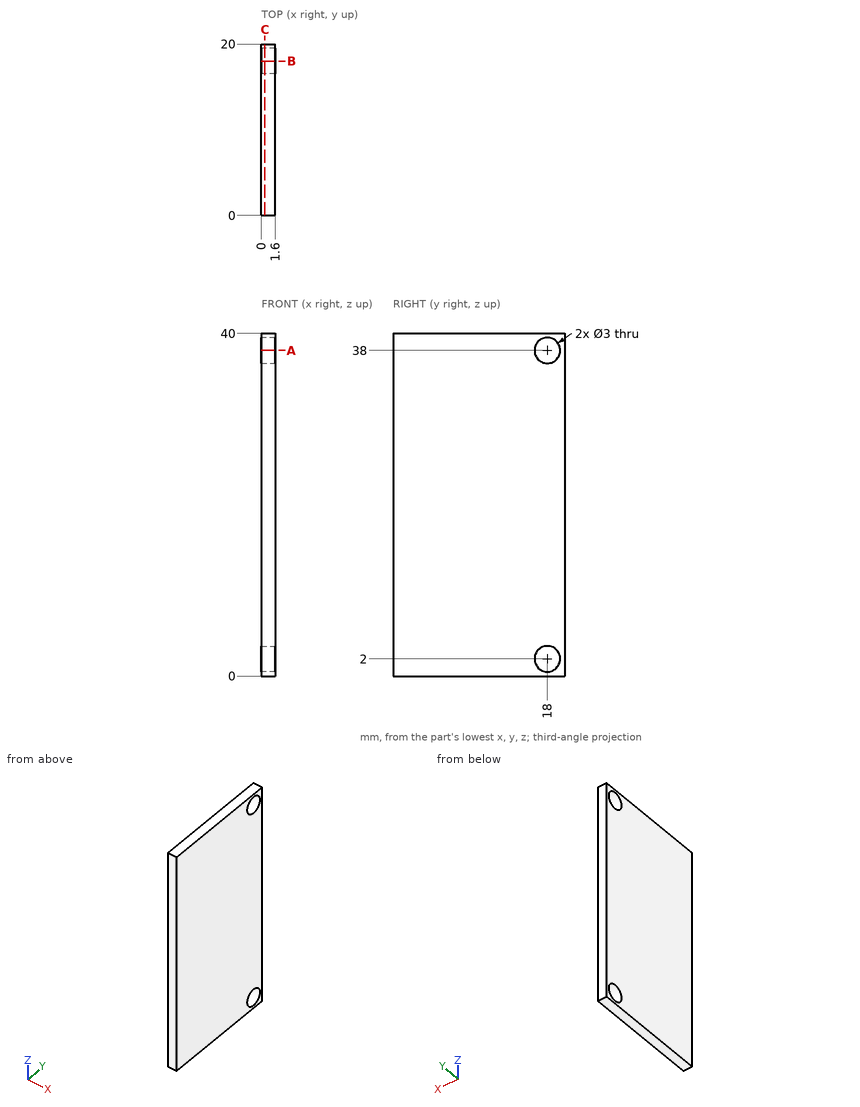
Check sheet for the drawn part. Datum: minimum x, y, z corner. Units: mm. Give positions to 0.01 mm unless a question says otherwise; leave off trailing zeros. Order: outer loops, then holes, each group sorted by start corner. A loop starts at its lowest first (then second) coordinate and runs counter-clockwise, first axis right, second up. Notation, with made-up numbers: (88.25, 33.25) - (115.25, 33.25) arc R26 cw to (115.25, 54.25) - close; hole circle Ø5 at (-8, 5). An arc over 180 degrees is marked (long way). Answer in a Markdown table with one row per item. Add a question column.
Q1. Material ranges on probe 1 along Y at (x, z) = (0.6, 2); probe 2 along Y at (x, z) = (0.8, 38.5), recorded low to high. Write a range as from..to.
Q2. Gauge pin test, flat end, axial feed: pin 1 (2.5 mm diameter, centred on y = 18, z = 2, fed in from -X). Record the tip position at first contact, or that the pin passes through.
Q3. Cross-section at C-C, the plane x = 0.4. Enter the section's corners in (y, z).
Q4. Cross-section at B-B, the plane y = 18. Enter the section's corners in (x, z), then the cut area to 3 significant figures.
Q5. Cross-section at A-A, the plane z = 38. Enter the section's corners in (x, y), then the cut area to 3 significant figures.
Check values:
| question | item | result |
|---|---|---|
| 1 | probe 1 | y = 0..16.5, 19.5..20 |
| 1 | probe 2 | y = 0..16.59, 19.41..20 |
| 2 | pin 1 | passes through |
| 3 | outline | (0, 0) - (20, 0) - (20, 40) - (0, 40) - close; hole circle Ø3 at (18, 2); hole circle Ø3 at (18, 38) |
| 4 | outline | (0, 0) - (1.6, 0) - (1.6, 0.5) - (0, 0.5) - close; (0, 3.5) - (1.6, 3.5) - (1.6, 36.5) - (0, 36.5) - close; (0, 39.5) - (1.6, 39.5) - (1.6, 40) - (0, 40) - close |
| 4 | area | 54.4 mm^2 |
| 5 | outline | (0, 0) - (1.6, 0) - (1.6, 16.5) - (0, 16.5) - close; (0, 19.5) - (1.6, 19.5) - (1.6, 20) - (0, 20) - close |
| 5 | area | 27.2 mm^2 |
